Read the model definition and answer for the solid it produces. Units are mm, in the model's axes. A direction names the side the tool comes from. Coordinates: 2 decimals unless noted, no trailing zeros. Loops run counter-clockwise (first coordinate to the right, second up) from the corner with the lowest first, then second, coordinate; pieces in that order, holes last. Notation, with made-up numbers: (78, 65) - (98, 65) arc R15 cw to (98, 85) - close; hole circle Ø2 at (28, -33). An arc over 180 degrees is marked (long way). One line per item, written item: value. Start each with the question number.
from build123d import *

# Parameters (mm, degrees)
F0_W      = 306.8140745163
F0_H      = 173.4216436744
F1_DEPTH  = 11.176
F3_DEPTH  = 52.324
F4_W      = 66.1161988974
F4_H      = 117.8840361536
F5_DEPTH  = 3.556
F7_DEPTH  = 43.942
F9_DEPTH  = 22.098
F10_W     = 20.6523872912
F10_H     = 88.7217707932
F11_DEPTH = 2.032
F12_W     = 14.7464126348
F12_H     = 22.3355772905
F13_DEPTH = 40.132
F15_DEPTH = 13.97
F17_DEPTH = 20.574
F19_DEPTH = 15.24
F21_DEPTH = 21.59
F22_W     = 51.9647672772
F22_H     = 55.9918135405
F23_DEPTH = 13.462
F24_R     = 10.9667117053
F25_DEPTH = 40.132
F26_R     = 5.0651062628
F27_DEPTH = 25.4


with BuildPart() as f1:
    # F0 (on Top) → F1 (new body)
    with BuildSketch(Plane.XY):
        with Locations((0.9204745293, 1.0380260646)):
            Rectangle(F0_W, F0_H)
    extrude(amount=F1_DEPTH)

    # F2 (on face) → F3 (join)
    with BuildSketch(Plane.XZ.offset(85.6727957726)):
        with BuildLine():
            ThreePointArc((0, 11.176), (-21.5048603714, 32.3440063265), (-43.0097207427, 11.176))
            Line((-43.0097207427, 11.176), (0, 11.176))
        make_face()
    extrude(amount=-F3_DEPTH)

    # F4 (on face) → F5 (join)
    with BuildSketch(Plane.XY.offset(11.176)):
        with Locations((73.4031423926, -26.7307776958)):
            Rectangle(F4_W, F4_H)
        Polygon((-42.968980968, 32.211240381), (40.345042944, 32.211240381), (106.4612418413, 32.211240381), (106.4612418413, 55.06047979), (-42.968980968, 55.06047979), align=None)
    extrude(amount=F5_DEPTH)

    # F6 (on face) → F7 (join)
    with BuildSketch(Plane.XY.offset(11.176)):
        Polygon((106.4612418413, 55.06047979), (106.4612418413, -85.6727957726), (154.3275117874, -85.6727957726), (154.3275117874, 87.7488479018), (-152.4865627289, 87.7488479018), (-152.4865627289, -85.6727957726), (-85.112079978, -85.6727957726), (-85.112079978, -18.8729763031), (-43.0097207427, -18.8729763031), (-42.968980968, 32.211240381), (-42.968980968, 55.06047979), align=None)
    extrude(amount=F7_DEPTH)

    # F8 (on face) → F9 (join)
    with BuildSketch(Plane.XZ.offset(-55.06047979)):
        Polygon((-42.968980968, 14.732), (31.7461304367, 14.732), (-42.968980968, 55.118), align=None)
    extrude(amount=F9_DEPTH)

    # F10 (on face) → F11 (join)
    with BuildSketch(Plane.XY.offset(55.118)):
        Polygon((-42.968980968, 33.5549861193), (-42.968980968, 55.06047979), (-152.4865627289, 55.06047979), (-152.4865627289, 33.5549861193), (-118.3801591396, 33.5549861193), (-97.7277718484, 33.5549861193), align=None)
        with Locations((-108.053965494, -10.8058992773)):
            Rectangle(F10_W, F10_H)
    extrude(amount=F11_DEPTH)

    # F12 (on face) → F13 (join)
    with BuildSketch(Plane.XY.offset(55.118)):
        with Locations((-133.7195262313, -18.4955450241)):
            Rectangle(F12_W, F12_H)
    extrude(amount=F13_DEPTH)

    # F14 (on face) → F15 (join)
    with BuildSketch(Plane.YZ.offset(-126.3463199139)):
        Polygon((-46.4369356632, 94.7568938136), (-29.6633336693, 75.184), (-29.6633336693, 95.25), align=None)
    extrude(amount=-F15_DEPTH)

    # F16 (on face) → F17 (join)
    with BuildSketch(Plane.XZ.offset(29.6633336693)):
        Polygon((-126.3463199139, 96.3086783886), (-126.3463199139, 75.184), (-113.2118999958, 96.3086783886), align=None)
    extrude(amount=-F17_DEPTH)

    # F18 (on face) → F19 (join)
    with BuildSketch(Plane(origin=(-141.0927325487, 0, 0), x_dir=(0, -1, 0), z_dir=(-1, 0, 0))):
        Polygon((7.3277563788, 75.184), (7.3277563788, 95.25), (-6.3867359422, 95.25), align=None)
    extrude(amount=-F19_DEPTH)

    # F20 (on face) → F21 (join)
    with BuildSketch(Plane(origin=(0, -7.3277563788, 0), x_dir=(-1, 0, 0), z_dir=(0, 1, 0))):
        Polygon((141.0927325487, 94.6096107364), (141.0927325487, 75.184), (156.4792990685, 94.6096107364), align=None)
    extrude(amount=-F21_DEPTH)

    # F22 (on face) → F23 (join)
    with BuildSketch(Plane.XY.offset(94.6096107364)):
        with Locations((-136.3664530218, -19.8239125311)):
            Rectangle(F22_W, F22_H)
    extrude(amount=F23_DEPTH)

    # F24 (on face) → F25 (join)
    with BuildSketch(Plane.XY.offset(108.0716107364)):
        with Locations((-126.7641037703, -12.5239156187)):
            Circle(F24_R)
    extrude(amount=F25_DEPTH)

    # F26 (on face) → F27 (join)
    with BuildSketch(Plane.XY.offset(148.2036107364)):
        with Locations((-126.7641037703, -12.5239156187)):
            Circle(F26_R)
    extrude(amount=F27_DEPTH)


solid = f1.part
1) Section D-D, the plane z = 135.5 is taken. Determine the outline of the cut face in (x, y).
2) Section A-A, the plane y = -39.5 is taken. Determine the outline of the cut face in (x, z).
3) Section B-B, the plane x = 48 is taken. Determine the outline of the cut face in (y, z).
4) Straight lines are drawn through the part: L1, parallel to X at y = 12, z = 31; L2, parallel to X at y = -76.5, z = 48; L3, parallel to Z at x = 9, y = -70. For each, find the intervals that lie inside material, in ascending order.
5) Flat-ended cylindrical pins translate along their axes: P1, Ø12, axis at y = 22.5, z = 38, coming from the -X side; P2, Ø0.6, axis at x = -81, z = 56, coming from the +Y side; P3, Ø3.5, axis at x = -117.5, z = 89.5, coming from the +Y side. Find the tip coordinate at first contact, or state that the pin passes through.
6) Section C-C, the plane y = 41 is taken. Determine the outline of the cut face in (x, z).
7) For faces 5 (the flat face through (-125.853, -4, 89)), 6 (the flat face through (-148.68, -17.97, 84.76)), 7 (the flat face through (-137, -47.82, 101)), determine the directions among +Z, -Z, +X, -X, +Y, -Y from which every point of the face is accessible in a straight line to the end or side of a thin tool.
8) Determine the mould class of faces 1 (the flat face through (-1, 2, 0)), 2 (the flat face through (-122, -15, 148.204)), 3 (the flat face through (-126.346, -19, 66)), 4 (the flat face through (-162.349, -20, 101)) for opening direction Z: released by +Z, released by -Z, zero draft, split by the parting line, or undercut.
Answer below:
1. outline: circle Ø21.93 at (-126.76, -12.52)
2. outline: (-162.35, 94.61) - (-140.32, 94.61) - (-140.32, 86.66) - (-126.35, 86.66) - (-126.35, 94.61) - (-110.38, 94.61) - (-110.38, 108.07) - (-162.35, 108.07) - close; (-152.49, 0) - (154.33, 0) - (154.33, 55.12) - (106.46, 55.12) - (106.46, 14.73) - (40.35, 14.73) - (40.35, 11.18) - (0, 11.18) arc R21.51 ccw to (-43.01, 11.18) - (-85.11, 11.18) - (-85.11, 55.12) - (-97.73, 55.12) - (-97.73, 57.15) - (-118.38, 57.15) - (-118.38, 55.12) - (-152.49, 55.12) - close
3. outline: (-85.67, 0) - (87.75, 0) - (87.75, 55.12) - (55.06, 55.12) - (55.06, 14.73) - (-85.67, 14.73) - close
4. L1: -152.49 to -42.99, 106.46 to 154.33
4. L2: -152.49 to -85.11, 106.46 to 154.33
4. L3: 0 to 11.18
5. P1: x = -152.49
5. P2: y = 55.06
5. P3: y = -9.09
6. outline: (-152.49, 0) - (154.33, 0) - (154.33, 55.12) - (106.46, 55.12) - (106.46, 14.73) - (31.75, 14.73) - (-42.97, 55.12) - (-42.97, 57.15) - (-152.49, 57.15) - close
7. face 5: +X, +Y
7. face 6: -X, +Y, -Y
7. face 7: +Z, +X, -X, -Y
8. face 1: released by -Z
8. face 2: released by +Z
8. face 3: undercut
8. face 4: zero draft
